Can you work these out from the model? Positions are in its coordinate system, mm. A direction names the side the tool comes from. Give positions to 0.01 mm unless a question says otherwise; leave off trailing zeros. Loops run counter-clockwise (first coordinate to the right, second up) from the corner with the lowest first, then second, coordinate; pieces in that order, holes last. Notation, with made-up numbers: (34, 51.25) - (41, 51.25) arc R17 cw to (41, 63.25) - close; hole circle Ø10 at (-17, 70). An arc over 180 degrees is marked (long way). Write item = value, one per line.
from build123d import *

# Parameters (mm, degrees)
SKETCH_1_R               = 11
EXTRUDE_1_DEPTH          = 68
CUT_EXTRUDE_START        = -19
SKETCH_2_R               = 11
SKETCH_2_R_2             = 10
CUT_EXTRUDE_1_DEPTH      = 19
CUT_EXTRUDE_2_DEPTH      = 70.756720106
CUT_EXTRUDE_2_DEPTH_BACK = 70.756720106
FILLET_1_R               = 0.5
SHELL_2_T                = -1
SKETCH_5_W               = 3
SKETCH_5_H               = 3
EXTRUDE_2_DEPTH          = 9


with BuildPart() as part:
    # Sketch 1 → Extrude 1 (new body)
    with BuildSketch(Plane(origin=(0, 0, 0), x_dir=(1, 0, 0), z_dir=(0, 1, 0))):
        with Locations(Location((0, 0, 0), (0, 0, 270))):
            Circle(SKETCH_1_R)
    extrude(amount=EXTRUDE_1_DEPTH)

    # Sketch 2 → Cut-Extrude 1 (cut)
    with BuildSketch(Plane(origin=(0, 68, 0), x_dir=(1, 0, 0), z_dir=(0, 1, 0)).offset(CUT_EXTRUDE_START)):
        with Locations(Location((0, 0, 0), (0, 0, 270))):
            Circle(SKETCH_2_R)
        with Locations(Location((0, 0, 0), (0, 0, 270))):
            Circle(SKETCH_2_R_2, mode=Mode.SUBTRACT)
    extrude(amount=CUT_EXTRUDE_1_DEPTH, mode=Mode.SUBTRACT)

    # Sketch 3 → Cut-Extrude 2 (cut, two sides: drawn at the far end of the back side and taken through both)
    with BuildSketch(Plane(origin=(0, 0, 0), x_dir=(0, 0, -1), z_dir=(1, 0, 0)).offset(-CUT_EXTRUDE_2_DEPTH_BACK)):
        Polygon((-10, 63), (10, 68), (-10, 68), align=None)
    extrude(amount=CUT_EXTRUDE_2_DEPTH + CUT_EXTRUDE_2_DEPTH_BACK, mode=Mode.SUBTRACT)

    # Fillet 1
    fillet_1_edges = [part.edges().sort_by_distance(p)[0] for p in [
        (10, 65.500000005, -2.1e-08),
    ]]
    fillet(fillet_1_edges, radius=FILLET_1_R)

    # Shell 2
    shell_2_openings = [part.faces().sort_by_distance(p)[0] for p in [
        (0, 0, 0),
    ]]
    offset(amount=SHELL_2_T, openings=shell_2_openings, kind=Kind.INTERSECTION)

    # Sketch 5 → Extrude 2 (add)
    with BuildSketch(Plane.XZ):
        with Locations((0, 12.397247359)):
            Rectangle(SKETCH_5_W, SKETCH_5_H)
    extrude(amount=-EXTRUDE_2_DEPTH)


solid = part.part
Q1. Imagine slicing it at C-C, the plane y = 39.5. Write out the boundary of the cut face in (x, z).
Output:
outline = circle Ø22 at (0, 0); hole circle Ø20 at (0, 0)
Q2. For pin 1 (12 mm diameter, centred on x = 8.5, y = 36, fed in from +Z); pin 2 (1.5 mm diameter, centred on y = 58, z = 2, fed in from +X); pin 3 (6 mm diameter, centred on x = 5, y = 51, fed in from +Z), each with a flat end and sliding along its axis, tell me the tip position at first contact or that it passes through.
Output:
pin_1 = 10.71
pin_2 = 9.92
pin_3 = 10.65
Q3. I need wall thicknesses on L1, parallel to Z at x = 0, y = 56.5; L2, parallel to X at y = 31, z = 0. Which ranges of each line are inside material? Lowest first, please.
Output:
L1 = -10 to -9, 9 to 10
L2 = -11 to -10, 10 to 11
Q4. Imagine slicing it at D-D, the plane y = 61. Write out the boundary of the cut face in (x, z).
Output:
outline = circle Ø20 at (0, 0); hole circle Ø18 at (0, 0)
Q5. Imagine slicing it at B-B, the plane z = 12.25. Write out the boundary of the cut face in (x, y).
Output:
outline = (-1.5, 0) - (1.5, 0) - (1.5, 9) - (-1.5, 9) - close
Q6. Imagine slicing it at A-A, the plane y = 5. Write out the boundary of the cut face in (x, z).
Output:
outline = (-1.5, 10.9) arc R11 ccw (long way) to (1.5, 10.9) - (1.5, 13.9) - (-1.5, 13.9) - close; hole circle Ø20 at (0, 0)
Q7. Which directions (+Z, -Z, +X, -X, +Y, -Y) give clear straight access to the entire face, cutting with the end or side of a thin tool? Please do faces 4 (the flat face through (2, 0, 10)), 5 (the flat face through (-10, 49, 2)), 6 (the flat face through (-1.5, 4, 12)), 7 (the flat face through (1.5, 4, 12)), 8 (the cylindrical face through (-9.76, 23.66, -2.17)).
Output:
face_4 = +Z, -Z, +X, -X, -Y
face_5 = +Y
face_6 = +Z, -X, +Y, -Y
face_7 = +Z, +X, +Y, -Y
face_8 = -Y
Q8. We'd pull the mould along Z, two halves only. Please class faces 1 (the flat face through (-0.147, 65.436, 0.254)), 2 (the flat face through (2, 48, -9)), 3 (the cylindrical face through (0, 56, -10)): released by +Z, released by -Z, zero draft, split by the parting line, or undercut.
Output:
face_1 = released by +Z
face_2 = undercut
face_3 = split by the parting line
